CAD build for the part. Positions are in the model's coordinates, mm. Face numbers are marked on the shaded views. A direction names the side the tool comes from. Coordinates: 2 decimals unless noted, no trailing zeros. Write each loop counter-clockwise with the first axis right and the second up, starting at its lowest first coordinate (ties: lowest second). Pieces come first, ordered by that corner, then holes. Notation, with made-up numbers: (74.25, -33) - (111.25, -33) arc R21 cw to (111.25, -16) - close; hole circle Ø2 at (-33.75, 44). An arc over 180 degrees is marked (long way). Answer in a Markdown table with one row per item. Add a question column.
Q1. Band-saw the part on B-B (x = 2). List the corners of the cut face in (y, z), and give its area (3 significant figures).
Q2. Band-saw the part on A-A (z = 0). State how many separate pieces and enclosed holes the cut face has, and give its area (4 significant figures).
Q3. Pin check, flat tips, straight feed: pin 1 (3 mm diameter, centred on x = 0, y = -2.5, fed in from +Z); pin 2 (5 mm diameter, centred on x = 2.5, z = -2.5, fed in from +Y). Stop position of each tip, or through.
Q4. Band-saw the part on D-D (x = -7.5). List the corners of the cut face in (y, z).
Q5. 3-axis set-ups, long thin cutter, end or side, ignore diameter. For the marked faces 1 and 2: which of +Z, -Z, +X, -X, +Y, -Y reach the whole face in a straight line?
Q6. Two-plate mould, pull along X, no slides. Class the marked faces 3, 4 and 5: +X half, -X half, draft (parallel to the pull), parting line (faces both ways), or undercut.
Q7. Drill centre lines: line 1 along X through (y, z) = (2.45, 0); line 2 along X through (y, z) = (-3.5, -1.25); line 3 along Z through (x, y) = (-6.5, 4). Where is each one in solid material? Low to high. Write a range as from..to.
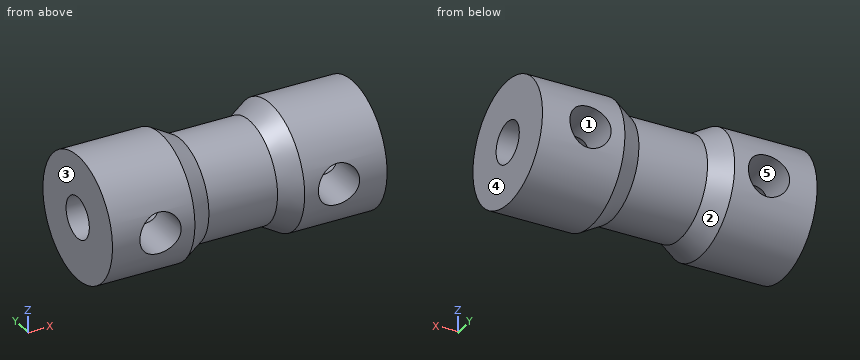
```python
from build123d import *

# Parameters (mm, degrees)
F2_R          = 1.5
F3_DEPTH      = 4.501
F3_DEPTH_BACK = 4.501
F4_R          = 1.5
F5_DEPTH      = 25
F5_DEPTH_BACK = 25


with BuildPart() as f1:
    # F0 (on Front) → F1 (revolve)
    with BuildSketch(Plane.XZ):
        Polygon((10, 0), (-10, 0), (-10, -4.5), (-4, -4.5), (-2.5, -3.65), (0, -3.65), (2.5, -3.65), (4, -4.5), (10, -4.5), align=None)
    revolve(axis=Axis((0, 0, 0), (1, 0, 0)))

    # F2 (on Front) → F3 (cut, two sides)
    with BuildSketch(Plane.XZ) as f3_sk:
        with Locations((-6.5, 0)):
            Circle(F2_R)
        with Locations((6.5, 0)):
            Circle(F2_R)
    extrude(amount=-F3_DEPTH, mode=Mode.SUBTRACT)
    extrude(f3_sk.sketch, amount=F3_DEPTH_BACK, mode=Mode.SUBTRACT)

    # F4 (on face) → F5 (cut, two sides)
    with BuildSketch(Plane.YZ.offset(10)) as f5_sk:
        Circle(F4_R)
    extrude(amount=-F5_DEPTH, mode=Mode.SUBTRACT)
    extrude(f5_sk.sketch, amount=F5_DEPTH_BACK, mode=Mode.SUBTRACT)


solid = f1.part
```
Checked values:
| question | item | result |
|---|---|---|
| 1 | outline | circle Ø7.3 at (0, 0); hole circle Ø3 at (0, 0) |
| 1 | area | 34.8 mm² |
| 2 | separate pieces | 6 |
| 2 | enclosed holes | 0 |
| 2 | area | 72.95 mm² |
| 3 | pin 1 | stops at z = 3.51 |
| 3 | pin 2 | stops at y = 4.47 |
| 4 | outline | (-4.36, -1.12) arc R4.5 ccw to (4.36, -1.12) - (1, -1.12) arc R1.5 cw to (-1, -1.12) - close; (-4.36, 1.12) - (-1, 1.12) arc R1.5 cw to (1, 1.12) - (4.36, 1.12) arc R4.5 ccw to start |
| 5 | face 1 | +Y, -Y |
| 5 | face 2 | none |
| 6 | face 3 | -X half |
| 6 | face 4 | +X half |
| 6 | face 5 | undercut |
| 7 | line 1 | x = -10..-8, -5..5, 8..10 |
| 7 | line 2 | x = -10..-7.33, -5.67..-2.62, 2.62..5.67, 7.33..10 |
| 7 | line 3 | z = -2.06..-1.5, 1.5..2.06 |
